Here's the drawing with two shaded views (mm, measured from the low corner). I have some questions. A direction names the side the tool comes from. Round coordinates to 2 decimals unless told otherwise and drop trailing zeros. Order: outer loops, then holes, each group sorted by start corner. A loop starts at its lowest first (then second) coordinate and runs counter-clockwise, first axis right, second up.
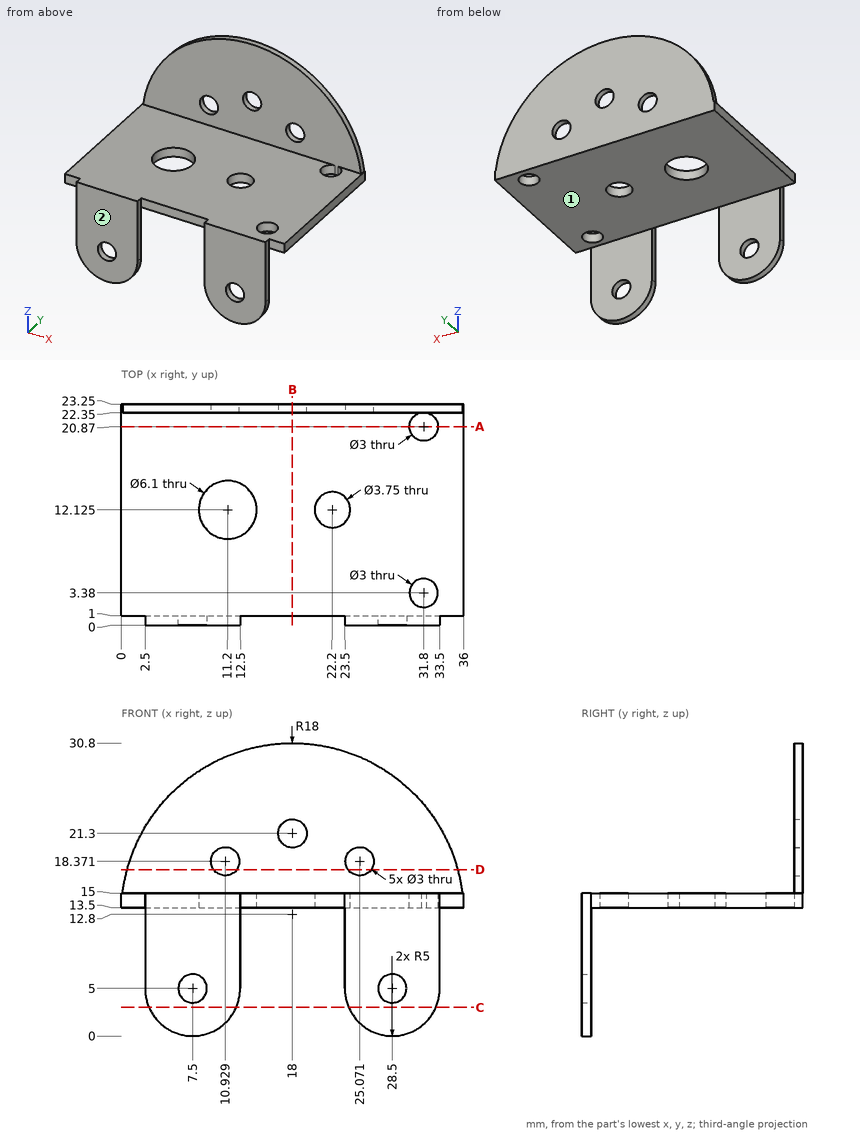
1. I need wall thicknesses on probe 1 along Z at (x, y) = (18.5, 14); probe 2 along Y at (x, z) = (32.5, 5.5); probe 3 along Y at (x, z) = (2, 18). Which ranges of each line are inside material? Lowest first, please.
Evaluation:
probe 1: z = 13.5 to 15
probe 2: y = 0 to 1
probe 3: y = 22.35 to 23.25
2. On a 3-axis mill with a long thin cutter (end or side, diameter ignored), from which of +Z, -Z, +X, -X, +Y, -Y can I reach the whole of each face in a straight line? I mean the marked faces 1 and 2. Say none if no direction works.
Evaluation:
face 1: -Z, +X, -X, +Y
face 2: +Z, -Z, +X, -X, -Y
3. I'm going to push flat-ended pins straight in: P1, Ø8, axis at x = 29, z = 7.5, coming from the +Y side; P2, Ø0.8, axis at y = 0.5, z = 9, coming from the -X side; P3, Ø2.5, axis at x = 31.8, y = 3.38, coming from the -Z side; P4, Ø4, axis at x = 21, z = 21.5, coming from the -Y side. Where does each tip first touch, or does it pass through?
Evaluation:
P1: stops at y = 1
P2: stops at x = 2.5
P3: passes through
P4: stops at y = 22.35
4. If we section it at A-A, the plane y = 20.87: Write out the boundary of the cut face in (x, z), and give its area (3 significant figures).
Evaluation:
outline: (0, 13.5) - (30.3, 13.5) - (30.3, 15) - (0, 15) - close; (33.3, 13.5) - (36, 13.5) - (36, 15) - (33.3, 15) - close
area: 49.5 mm2
5. If we section it at D-D, the plane z = 17.5: Write out the boundary of the cut face in (x, y).
Evaluation:
outline: (0.62, 22.35) - (9.71, 22.35) - (9.71, 23.25) - (0.62, 23.25) - close; (12.15, 22.35) - (23.85, 22.35) - (23.85, 23.25) - (12.15, 23.25) - close; (26.29, 22.35) - (35.38, 22.35) - (35.38, 23.25) - (26.29, 23.25) - close
6. If we section it at C-C, the plane z = 3: Write out the boundary of the cut face in (x, y).
Evaluation:
outline: (2.92, 0) - (12.08, 0) - (12.08, 1) - (2.92, 1) - close; (23.92, 0) - (33.08, 0) - (33.08, 1) - (23.92, 1) - close
7. If we section it at B-B, the plane x = 18: Write out the boundary of the cut face in (y, z), and give its area (3 significant figures).
Evaluation:
outline: (1, 13.5) - (23.25, 13.5) - (23.25, 19.8) - (22.35, 19.8) - (22.35, 15) - (1, 15) - close; (22.35, 22.8) - (23.25, 22.8) - (23.25, 30.8) - (22.35, 30.8) - close
area: 44.9 mm2
